```python
from build123d import *

# Parameters (mm, degrees)
SKETCH_1_R          = 3.1
SKETCH_1_R_2        = 24
EXTRUDE_1_DEPTH     = 5
SKETCH_2_R          = 1.6
CUT_EXTRUDE_1_DEPTH = 44
CUT_EXTRUDE_2_DEPTH = 34
FILLET_1_R          = 3
CUT_EXTRUDE_3_DEPTH = 34
FILLET_2_R          = 3


with BuildPart() as part:
    # 草图1 → 凸台-拉伸1 (new body)
    with BuildSketch(Plane.XY):
        with BuildLine():
            Line((-103.589105886, 32.89722268), (-14.961918346, 56.036814298))
            ThreePointArc((-14.961918346, 56.036814298), (-9.057902271, 55.29071215), (-5.302552139, 50.674282835))
            Line((-5.302552139, 50.674282835), (9.548000145, 2.9724894))
            ThreePointArc((9.548000145, 2.9724894), (8.743053177, -4.853763606), (2.526315789, -9.675625485))
            Line((2.526315789, -9.675625485), (-86.410526316, -32.89712665))
            ThreePointArc((-86.410526316, -32.89712665), (-127.897174666, -8.589289785), (-103.589105886, 32.89722268))
        make_face()
        Circle(SKETCH_1_R, mode=Mode.SUBTRACT)
        with Locations((-95, 0)):
            Circle(SKETCH_1_R_2, mode=Mode.SUBTRACT)
        with Locations((-12.940952255, 48.296291314)):
            Circle(SKETCH_1_R, mode=Mode.SUBTRACT)
    extrude(amount=EXTRUDE_1_DEPTH)

    # 草图2 → 切除-拉伸1 (cut)
    with BuildSketch(Plane(origin=(0, 0, 0), x_dir=(-1, 0, 0), z_dir=(0, 0, -1))):
        with Locations((21.238501013, -11.746543996)):
            Circle(SKETCH_2_R)
        with Locations((46.395127275, -18.314965049)):
            Circle(SKETCH_2_R)
        with Locations((71.551753537, -24.883386101)):
            Circle(SKETCH_2_R)
        with Locations((95, -30)):
            Circle(SKETCH_2_R)
        with Locations((125, 0)):
            Circle(SKETCH_2_R)
        with Locations((95, 30)):
            Circle(SKETCH_2_R)
        with Locations((71.274432107, 26.380963088)):
            Circle(SKETCH_2_R)
        with Locations((45.645838312, 22.002015719)):
            Circle(SKETCH_2_R)
        with Locations((20.017244516, 17.623068351)):
            Circle(SKETCH_2_R)
    extrude(amount=-CUT_EXTRUDE_1_DEPTH, mode=Mode.SUBTRACT)

    # 草图3 → 切除-拉伸2 (cut)
    with BuildSketch(Plane(origin=(0, 0, 0), x_dir=(-1, 0, 0), z_dir=(0, 0, -1))):
        with BuildLine():
            Line((70.381933652, -20.443845267), (8.974874995, -4.410398942))
            ThreePointArc((8.974874995, -4.410398942), (8.011191904, 5.985048394), (-1.684210526, 9.85715146))
            Line((-1.684210526, 9.85715146), (72.232775022, 22.486739799))
            ThreePointArc((72.232775022, 22.486739799), (63.029697498, 1.378317076), (70.381933652, -20.443845267))
        make_face()
    extrude(amount=-CUT_EXTRUDE_2_DEPTH, mode=Mode.SUBTRACT)

    # 圆角1
    fillet_1_edges = [part.edges().sort_by_distance(p)[0] for p in [
        (-8.974874995, -4.410398942, 2.5),
        (1.684210526, 9.85715146, 2.5),
        (-72.232775022, 22.486739799, 2.5),
        (-70.381933652, -20.443845267, 2.5),
    ]]
    fillet(fillet_1_edges, radius=FILLET_1_R)

    # 草图4 → 切除-拉伸3 (cut)
    with BuildSketch(Plane(origin=(0, 0, 0), x_dir=(-1, 0, 0), z_dir=(0, 0, -1))):
        Polygon((20.689823209, 46.27314566), (77.356433109, 31.478112128), (12.641453143, 20.420794919), align=None)
    extrude(amount=-CUT_EXTRUDE_3_DEPTH, mode=Mode.SUBTRACT)

    # 圆角2
    fillet_2_edges = [part.edges().sort_by_distance(p)[0] for p in [
        (-12.641453143, 20.420794919, 2.5),
        (-20.689823209, 46.27314566, 2.5),
        (-77.356433109, 31.478112128, 2.5),
    ]]
    fillet(fillet_2_edges, radius=FILLET_2_R)


solid = part.part
```
Geometry check sheet. Reference: the model listing, model coordinates, mm. A direction names the side the tool comes from. Coordinates: 2 decimals unless noted, no trailing zeros. Loops run counter-clockwise (first coordinate to the right, second up) from the corner with the lowest first, then second, coordinate; pieces in that order, holes last.
Item 1: Sectioned sample at A-A, the plane y = 0. Record the boundary of the cut face in (x, z).
Item 2: Sectioned sample at D-D, the plane x = -95. Record the boundary of the cut face in (y, z).
Item 3: Go/stop test with flat-tipped pins: pin 1 Ø5 at (x, y) = (-95, -30) entering from -Z; pin 2 Ø1 at (x, z) = (-83, 2.5) entering from -Y; pin 3 Ø1.9 at (x, y) = (-71.27, 26.38) entering from -Z; pin 4 Ø2 at (y, z) = (22.5, 3.5) entering from -X. Record where each tip stops, or that it passes through.
Item 4: Thickness scan on line 1 (Y direction, x = -47, z = 3.95); line 2 (X direction, y = -4, z = 1.25); line 3 (X direction, y = -1, z = 2). Record the ranges inside material, lowest first.
Item 5: Sectioned sample at B-B, the plane x = -125. Record the boundary of the cut face in (y, z).
Item 6: Access from +Z, -Z, +X, -X, +Y, -Y to the whole of each face (thin tool, end or side, straight path). Record for faces 5 (the face through (-59, 22, 5)), 6 (the face through (-10.25, -3.9, 2.54)).
Item 7: Sectioned sample at C-C, the plane z = 2.2. Count the separate pieces of the cut face and the enclosed holes in it, then the cut area to 3 significant figures.
Item 8: Release check for a two-part mould opening along X. For faces 1 (the face through (-59.896, 44.305, 2.465)), 2 (the face through (-59, 22, 0)), 3 (the face through (-6.798, 9.765, 2.535)), 4 (the face through (-13.34, 51.37, 2.46)) record: released by +X, released by -X, zero draft, split by the parting line, or undercut.
Check result:
1. outline: (-129, 0) - (-126.6, 0) - (-126.6, 5) - (-129, 5) - close; (-123.4, 0) - (-119, 0) - (-119, 5) - (-123.4, 5) - close; (-71, 0) - (-63, 0) - (-63, 5) - (-71, 5) - close; (-10, 0) - (-3.1, 0) - (-3.1, 5) - (-10, 5) - close; (3.1, 0) - (10, 0) - (10, 5) - (3.1, 5) - close
2. outline: (-34, 0) - (-31.6, 0) - (-31.6, 5) - (-34, 5) - close; (-28.4, 0) - (-24, 0) - (-24, 5) - (-28.4, 5) - close; (24, 0) - (28.4, 0) - (28.4, 5) - (24, 5) - close; (31.6, 0) - (35.14, 0) - (35.14, 5) - (31.6, 5) - close
3. pin 1: stops at z = 0
3. pin 2: stops at y = -32.14
3. pin 3: passes through
3. pin 4: stops at x = -121.34
4. line 1: y = -22.61 to -19.8, -16.83 to -14.34, 18.18 to 21.15, 22.85 to 26.29, 39.4 to 47.67
4. line 2: x = -128.76 to -118.66, -71.34 to -63.25, -10.32 to 9.17
4. line 3: x = -128.99 to -126.25, -123.75 to -118.98, -71.02 to -63.02, -9.95 to -2.93, 2.93 to 9.95
5. outline: (-16, 0) - (-1.6, 0) - (-1.6, 5) - (-16, 5) - close; (1.6, 0) - (16, 0) - (16, 5) - (1.6, 5) - close
6. face 5: +Z, +X, -X, +Y, -Y
6. face 6: +Z, -Z
7. separate pieces: 1
7. enclosed holes: 14
7. area: 4,360 mm2
8. face 1: released by -X
8. face 2: zero draft
8. face 3: undercut
8. face 4: undercut
